Could you check a few things on this model? Use its own coordinates, in mm. A direction names the side the tool comes from. Round coordinates to 2 decimals unless told otherwise and drop trailing zeros. Loops run counter-clockwise (first coordinate to the right, second up) from the corner with the lowest first, then second, coordinate; pieces in that order, holes last. Notation, with made-up numbers: M 36,34 L 54,34 A34 ccw 54,69 Z; hole C 18,25 d9. An arc over 180 degrees is marked long. One line per item, written item: value. Start each with the question number.
Q1. Imagine slicing it at C-C (z = 7.5). Please give me the cut outline in (x, y), then the cut area to 3 significant figures.
Q2. Thinking about a two-plate mould opening in X: for faces 1 (the face through (6.59, -0.13, -1.46)), 2 (the face through (-9.7, 10.5, -1.25)), 3 (the face through (7.48, -10.014, 12.223)), which applies, released by +X, released by -X, zero draft, split by the parting line, or undercut?
Q3. I'm going to push flat-ended pins straight in: pin 1 Ø2 at (x, z) = (7, 0) entering from +Y; pin 2 Ø5 at (y, z) = (-5, 11.5) entering from +X; pin 3 Ø1.1 at (x, y) = (11, 10.5) entering from -Z; pin 4 Ø1 at (x, z) = (3.5, -8.5) entering from -Y. Where does each tip first touch, or does it pass through?
Q4. Which directions (+Z, -Z, +X, -X, +Y, -Y) give clear straight access to the entire face, cutting with the end or side of a thin tool? Please do faces 4 (the face through (3.1, -9, -6.5)), 5 (the face through (-10, 10, 0)), 6 (the face through (-0.2, 10.5, -7.75)), 7 (the face through (0, 11, 8)).
Q5. Imagine slicing it at D-D (y = -8). Please give me the cut outline in (x, z), then the cut area to 3 significant figures.
Q6. Please list where these lines run through material, in increasing order: line 1 along Z through (x, y) = (0, -10.4); line 2 along Y through (x, z) = (-4.25, -7.75); line 3 along Y through (x, z) = (5, 5).
Q7. Imagine slicing it at B-B (x = -0.5). Please give me the cut outline in (y, z).
Q8. Imagine slicing it at A-A (z = 0). Please give me the cut outline in (x, y).
from build123d import *

# Parameters (mm, degrees)
CUT_EXTRUDE2_DEPTH      = 1
CUT_EXTRUDE3_DEPTH      = 17
CUT_EXTRUDE3_DEPTH_BACK = 1
CUT_EXTRUDE3_START      = -40
SKETCH5_W               = 42.611665196
SKETCH5_H               = 2.5
SKETCH3_R               = 1.25
CUT_EXTRUDE1_DEPTH      = 9.5


with BuildPart() as part:
    # Sketch2 → Revolve1 (revolve)
    with BuildSketch(Plane(origin=(0, 0, 0), x_dir=(0, 0, -1), z_dir=(1, 0, 0))):
        Polygon((-15, 11), (-15, 9), (-6.75, 9), (-6.75, -9), (-15, -9), (-15, -11), (-8.5, -11), (-8.5, -13), (-4.5, -13), (-4.5, -12), (-4.5, 11), align=None)
    revolve(axis=Axis((0, 15.5, 0), (0, -1, 0)))

    # Sketch4 → Cut-Extrude2 (cut)
    with BuildSketch(Plane(origin=(0, 11, 0), x_dir=(1, 0, 0), z_dir=(0, 1, 0))):
        Polygon((-2.25827734, 9.25), (1.74172266, 9.25), (1.74172266, 11.500000233), (4.74172266, 8.5), (1.74172266, 5.500000233), (1.74172266, 7.75), (-2.25827734, 7.75), align=None)
    extrude(amount=-CUT_EXTRUDE2_DEPTH, mode=Mode.SUBTRACT)

    # Sketch5 → Cut-Extrude3 (cut, two sides: drawn at the far end of the back side and taken through both)
    with BuildSketch(Plane.XZ.offset(13).offset(CUT_EXTRUDE3_START - CUT_EXTRUDE3_DEPTH_BACK)):
        Rectangle(SKETCH5_W, SKETCH5_H)
    extrude(amount=CUT_EXTRUDE3_DEPTH + CUT_EXTRUDE3_DEPTH_BACK, mode=Mode.SUBTRACT)

    # Sketch3 → Cut-Extrude1 (cut, symmetric)
    with BuildSketch(Plane.XZ.offset(11)):
        with Locations(Location((0, 8, 0), (0, 0, 270))):
            Circle(SKETCH3_R)
        with Locations(Location((7.425425002, 10.973858189, 0), (0, 0, 270))):
            Circle(SKETCH3_R)
    extrude(amount=CUT_EXTRUDE1_DEPTH, both=True, mode=Mode.SUBTRACT)


solid = part.part
Report:
1. outline: M -12.99,-11 L -4,-11 L -4,-13 L -1.15,-13 L -1.15,-9 L -12.99,-9 Z; M -12.99,9 L 12.99,9 L 12.99,11 L -12.99,11 Z; M 1.15,-13 L 4,-13 L 4,-11 L 12.99,-11 L 12.99,-9 L 1.15,-9 Z
1. area: 111 mm²
2. face 1: split by the parting line
2. face 2: zero draft
2. face 3: undercut
3. pin 1: stops at y = 10
3. pin 2: passes through
3. pin 3: stops at z = -10.76
3. pin 4: stops at y = -11
4. face 4: none
4. face 5: +X, -X, +Y
4. face 6: +Y
4. face 7: +Z, -Z, +X, -X, +Y
5. outline: C 0,0 d13.5; hole C 0,0 d9
5. area: 79.5 mm²
6. line 1: z = -15 to -4.5, 4.5 to 6.75, 9.25 to 15
6. line 2: y = -11 to -9, 9 to 11
6. line 3: y = -13 to -9, 9 to 11
7. outline: M -13,-8.49 L -11,-8.49 L -11,-14.99 L -9,-14.99 L -9,-6.73 L 9,-6.73 L 9,-14.99 L 11,-14.99 L 11,-9.25 L 10,-9.25 L 10,-7.75 L 11,-7.75 L 11,-4.47 L -13,-4.47 Z; M -13,4.47 L 11,4.47 L 11,14.99 L 9,14.99 L 9,6.73 L -9,6.73 L -9,6.85 L -13,6.85 Z; M -11,9.15 L -9,9.15 L -9,14.99 L -11,14.99 Z
8. outline: M -15,-11 L -8.5,-11 L -8.5,-13 L -4.5,-13 L -4.5,10 L -15,10 L -15,9 L -6.75,9 L -6.75,-9 L -15,-9 Z; M 4.5,-13 L 8.5,-13 L 8.5,-11 L 15,-11 L 15,-9 L 6.75,-9 L 6.75,9 L 15,9 L 15,10 L 4.5,10 Z
